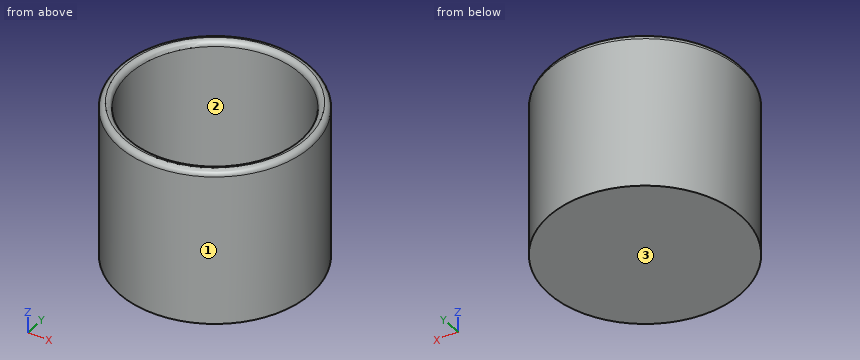
from build123d import *

# Parameters (mm, degrees)
F1_R = 22.4423927589
F3_T = -2.54
F4_R = 1.26999


# Not quite as in the source:
# - a fillet or chamfer is up to 0.001 mm smaller than in the source, because OpenCascade refuses the exact size


with BuildPart() as f2:
    # F2: sweep along a path in F0
    with BuildLine(Plane.XZ) as f2_path:
        Line((-22.9121223092, 36.5854799747), (-22.9121223092, 0))
    # F1 (on Top) → F2 (sweep)
    with BuildSketch(Plane.XY):
        Circle(F1_R)
    sweep(path=f2_path.line)

    # F3
    f3_openings = [f2.faces().sort_by_distance(p)[0] for p in [
        (0, 0, 36.58548),
    ]]
    offset(amount=F3_T, openings=f3_openings)

    # F4 (radius 1.27 in the source; OpenCascade refuses exactly that, so slightly less here)
    f4_edges = [f2.edges().sort_by_distance(p)[0] for p in [
        (-22.442393, 0, 36.58548),
        (-19.902393, 0, 36.58548),
    ]]
    fillet(f4_edges, radius=F4_R)


solid = f2.part
Design review of the part built by this model. Coordinates are the model's own, in mm. Face numbers are marked on the shaded views. Coordinates: 2 decimals unless noted, no trailing zeros. Write each loop counter-clockwise with the first axis right and the second up, starting at its lowest first coordinate (ties: lowest second). Pieces come first, ordered by that corner, then holes. Notation, with made-up numbers: (35, 57) -> (46, 57) arc R12 cw to (46, 66) -> close; hole circle Ø2 at (82, 73.25). An arc over 180 degrees is marked (long way). Write each question's results on one line, items separated by ' | '. Start each with the question number.
(1) The part is to be moulded in two halves that separate along X. For the marked faces 1, 2 and 3, say which applies: pulls with the +X half, pulls with the -X half, needs draft (parallel to the pull), parting line crosses it, or undercut.
(2) Clearance check with flat-ended pins moving along their axes: P1, Ø1.5, axis at x = -9, z = 4, coming from the -Y side; P2, Ø1.5, axis at x = -16.5, z = 22.5, coming from the +Y side; P3, Ø8, axis at x = 3.5, z = 6, coming from the -Y side; P4, Ø5, axis at x = 5.5, y = -16.5, coming from the -Z side. State where each tip first meets the part, or that it passes through.
(3) For line 1 along X through (y, z) = (0, 27); line 2 along Z through (x, y) = (15.5, 3), list the stretches that pass through material, from the lowest coordinate up. Write a range as from..to.
(4) Take a section at B-B on z = 32.5. Write out the cut boundary in (x, y), and give its area (3 significant figures).
Results found:
1) face 1: parting line crosses it | face 2: undercut | face 3: needs draft
2) P1: stops at y = -20.87 | P2: stops at y = 15.99 | P3: stops at y = -22.44 | P4: stops at z = 0
3) line 1: x = -22.44..-19.9, 19.9..22.44 | line 2: z = 0..2.54
4) outline: circle Ø44.88 at (0, 0); hole circle Ø39.8 at (0, 0) | area: 338 mm2
